from build123d import *

# Parameters (mm, degrees)
SKETCH1_R           = 1.1
SKETCH1_R_2         = 1.05
SKETCH1_R_3         = 2
BOSS_EXTRUDE1_DEPTH = 1.9
SKETCH2_W           = 20
SKETCH2_H           = 18
SKETCH2_R           = 1.1
SKETCH2_R_2         = 1.05
SKETCH2_R_3         = 1
BOSS_EXTRUDE2_DEPTH = 1


with BuildPart() as part:
    # Sketch1 → Boss-Extrude1 (new body)
    with BuildSketch(Plane.XY):
        Polygon((-10, 9), (10, 9), (10, -9), (-10, -9), (-10, -1.1), (-10, 4), align=None)
        with Locations(Location((7.5, -6.5, 0), (0, 0, 180))):
            Circle(SKETCH1_R, mode=Mode.SUBTRACT)
        with Locations(Location((-7.5, 6.5, 0), (0, 0, 180))):
            Circle(SKETCH1_R, mode=Mode.SUBTRACT)
        with Locations(Location((-8.05, -6.825, 0), (0, 0, 180))):
            Circle(SKETCH1_R_2, mode=Mode.SUBTRACT)
        with Locations(Location((7.5, 6.5, 0), (0, 0, 180))):
            Circle(SKETCH1_R_2, mode=Mode.SUBTRACT)
        with Locations(Location((-4.05, -4.65, 0), (0, 0, 180))):
            Circle(SKETCH1_R_3, mode=Mode.SUBTRACT)
    extrude(amount=BOSS_EXTRUDE1_DEPTH)

    # Sketch2 → Boss-Extrude2 (add)
    with BuildSketch(Plane.XY.offset(1.9)):
        Rectangle(SKETCH2_W, SKETCH2_H)
        with Locations(Location((-7.5, 6.5, 0), (0, 0, 180))):
            Circle(SKETCH2_R, mode=Mode.SUBTRACT)
        with Locations(Location((7.5, 6.5, 0), (0, 0, 180))):
            Circle(SKETCH2_R_2, mode=Mode.SUBTRACT)
        with Locations(Location((7.5, -6.5, 0), (0, 0, 180))):
            Circle(SKETCH2_R, mode=Mode.SUBTRACT)
        with Locations(Location((-8.05, -6.825, 0), (0, 0, 180))):
            Circle(SKETCH2_R_2, mode=Mode.SUBTRACT)
        with Locations((-4.05, -4.65)):
            Circle(SKETCH2_R_3, mode=Mode.SUBTRACT)
    extrude(amount=BOSS_EXTRUDE2_DEPTH)


solid = part.part
For this review, take the finished solid that the model builds, in its own axes (mm). A direction names the side the tool comes from. Round coordinates to 2 decimals unless told otherwise and drop trailing zeros. Loops run counter-clockwise (first coordinate to the right, second up) from the corner with the lowest first, then second, coordinate; pieces in that order, holes last. Notation, with made-up numbers: (-40, 10) - (-20, 10) arc R27 ccw to (-20, 27) - close; hole circle Ø4 at (80, -23). An arc over 180 degrees is marked (long way). One line per question, with ' | ' between items.
Q1. For pin 1 (1.2 mm diameter, centred on x = -5, y = -4, fed in from -Z); pin 2 (3.5 mm diameter, centred on x = 7.5, y = -6.5, fed in from -Z), all flat-tipped, find the tip position at first contact; note any pin that passes through.
Taken from the geometry:
pin 1: stops at z = 1.9 | pin 2: stops at z = 0
Q2. The part is to be moulded in two halves that separate along Y. For faces 1 (the cylindrical face through (-8.53, -5.89, 1.43)), 2 (the flat face through (-10, 0, 1)), 3 (the flat face through (0, 9, 1)), say which applies: released by +Y, released by -Y, zero draft, split by the parting line, or undercut.
Taken from the geometry:
face 1: undercut | face 2: zero draft | face 3: released by +Y
Q3. Take a section at D-D (z = 2.4). Give the boundary of the cut face in (x, y) (3 decimals).
Taken from the geometry:
outline: (-10, -9) - (10, -9) - (10, 9) - (-10, 9) - close; hole circle Ø2.1 at (-8.05, -6.825); hole circle Ø2.2 at (-7.5, 6.5); hole circle Ø2 at (-4.05, -4.65); hole circle Ø2.2 at (7.5, -6.5); hole circle Ø2.1 at (7.5, 6.5)
Q4. Take a section at C-C (y = -4.65). Give the boundary of the cut face in (x, z), and give its area (3 significant figures).
Taken from the geometry:
outline: (-10, 0) - (-6.05, 0) - (-6.05, 1.9) - (-5.05, 1.9) - (-5.05, 2.9) - (-10, 2.9) - close; (-3.05, 1.9) - (-2.05, 1.9) - (-2.05, 0) - (10, 0) - (10, 2.9) - (-3.05, 2.9) - close | area: 48.4 mm²
Q5. For line 1 along X through (y, z) = (6.5, 1.35); line 2 along Y through (x, z) = (7.5, 1); line 3 along X through (y, z) = (-4.65, 1.3), list the stretches that pass through material, from the lowest coordinate up. Write a range as [from, to].
Taken from the geometry:
line 1: x = [-10, -8.6], [-6.4, 6.45], [8.55, 10] | line 2: y = [-9, -7.6], [-5.4, 5.45], [7.55, 9] | line 3: x = [-10, -6.05], [-2.05, 10]
Q6. Tool access review of faces 4 (the flat face through (0, 0, 0)), 5 (the cylindrical face through (-5.958, -5.251, 0.937)): name each direction out of +Z, -Z, +X, -X, +Y, -Y from which nothing blocks a thin tool from reaching the whole face with its end or side.
Taken from the geometry:
face 4: -Z, +X, -X, +Y, -Y | face 5: -Z
Q7. Take a section at A-A (y = 6.5). Give the boundary of the cut face in (x, z), and give its area (3 significant figures).
Taken from the geometry:
outline: (-10, 0) - (-8.6, 0) - (-8.6, 2.9) - (-10, 2.9) - close; (-6.4, 0) - (6.45, 0) - (6.45, 2.9) - (-6.4, 2.9) - close; (8.55, 0) - (10, 0) - (10, 2.9) - (8.55, 2.9) - close | area: 45.5 mm²
Q8. Take a section at B-B (x = -4.05). Give the boundary of the cut face in (y, z).
Taken from the geometry:
outline: (-9, 0) - (-6.65, 0) - (-6.65, 1.9) - (-5.65, 1.9) - (-5.65, 2.9) - (-9, 2.9) - close; (-3.65, 1.9) - (-2.65, 1.9) - (-2.65, 0) - (9, 0) - (9, 2.9) - (-3.65, 2.9) - close
